The listing builds one solid part. Answer for the finished solid, in the listing's coordinates (mm). Give positions to 0.01 mm unless a question says otherwise; leave off trailing zeros. Order: outer loops, then holes, each group sorted by start corner. A loop starts at its lowest first (then second) coordinate and runs counter-clockwise, first axis right, second up. Notation, with made-up numbers: (75.25, -17.75) - (83.25, -17.75) arc R28 ccw to (83.25, 1.25) - close; hole circle Ø10 at (-24, -29.5). An arc over 180 degrees is marked (long way). Answer in a Markdown table with one row per item.
from build123d import *

# Parameters (mm, degrees)
SKETCH1_W           = 145
SKETCH1_H           = 68
BOSS_EXTRUDE1_DEPTH = 2
SKETCH2_R           = 1.65
SKETCH2_R_2         = 3
SKETCH2_R_3         = 1.1
CUT_EXTRUDE1_DEPTH  = 81.101498113


with BuildPart() as part:
    # Sketch1 → Boss-Extrude1 (new body)
    with BuildSketch(Plane.XY):
        Rectangle(SKETCH1_W, SKETCH1_H)
    extrude(amount=BOSS_EXTRUDE1_DEPTH)

    # Sketch2 → Cut-Extrude1 (cut, through all)
    with BuildSketch(Plane.XY.offset(2)):
        with Locations((53, 20)):
            Circle(SKETCH2_R)
        with Locations((53, -20)):
            Circle(SKETCH2_R)
        with Locations((-59.5, 15)):
            Circle(SKETCH2_R_2)
        with Locations((-59.5, -15)):
            Circle(SKETCH2_R_2)
        with Locations((-59.5, 0)):
            Circle(SKETCH2_R_3)
        with BuildLine():
            Line((61.5, -13.5), (44.5, -13.5))
            ThreePointArc((44.5, -13.5), (43.792893219, -13.207106781), (43.5, -12.5))
            Line((43.5, -12.5), (43.5, 12.5))
            ThreePointArc((43.5, 12.5), (43.792893219, 13.207106781), (44.5, 13.5))
            Line((44.5, 13.5), (61.5, 13.5))
            ThreePointArc((61.5, 13.5), (62.207106781, 13.207106781), (62.5, 12.5))
            Line((62.5, 12.5), (62.5, -12.5))
            ThreePointArc((62.5, -12.5), (62.207106781, -13.207106781), (61.5, -13.5))
        make_face()
    extrude(amount=-CUT_EXTRUDE1_DEPTH, mode=Mode.SUBTRACT)


solid = part.part
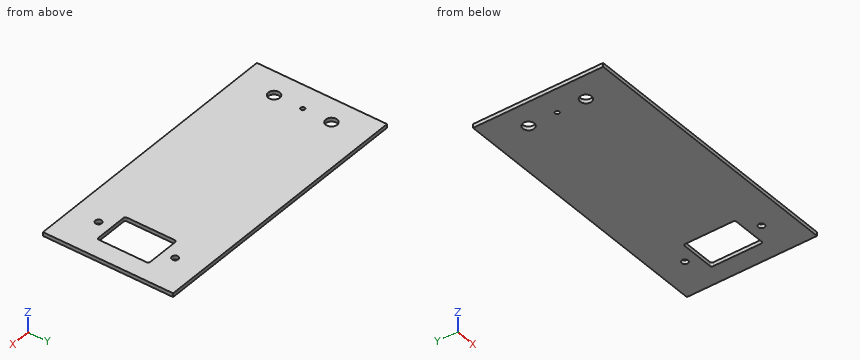
Item 1: Find section A-A on y = -9. Write down the section's boundary in (x, z).
Answer block:
| item | result |
|---|---|
| outline | (-72.5, 0) - (43.5, 0) - (43.5, 2) - (-72.5, 2) - close; (62.5, 0) - (72.5, 0) - (72.5, 2) - (62.5, 2) - close |
Item 2: This flat-tipped pin is pushed along its axis until it touches: P1, Ø5.5, axis at x = -59.5, y = 15, coming from the +Z side. Where does it stop, or does it pass through?
Answer block:
| item | result |
|---|---|
| P1 | through |
Item 3: Find section B-B on x = 53. Write down the section's boundary in (y, z), then the cut area to 3 significant figures.
Answer block:
| item | result |
|---|---|
| outline | (-34, 0) - (-21.65, 0) - (-21.65, 2) - (-34, 2) - close; (-18.35, 0) - (-13.5, 0) - (-13.5, 2) - (-18.35, 2) - close; (13.5, 0) - (18.35, 0) - (18.35, 2) - (13.5, 2) - close; (21.65, 0) - (34, 0) - (34, 2) - (21.65, 2) - close |
| area | 68.8 mm² |
Item 4: Find section C-C on y = -20. Write down the section's boundary in (x, z), then the cut area to 3 significant figures.
Answer block:
| item | result |
|---|---|
| outline | (-72.5, 0) - (51.35, 0) - (51.35, 2) - (-72.5, 2) - close; (54.65, 0) - (72.5, 0) - (72.5, 2) - (54.65, 2) - close |
| area | 283 mm² |
Item 5: Consider line 1 (Y direction, x = 53, z = 0.95); line 2 (Y direction, x = -59.5, z = 0.5); line 3 (X direction, y = -10.5, z = 0.4). Determine where each line is inside the solid, lowest interval first.
Answer block:
| item | result |
|---|---|
| line 1 | -34 to -21.65, -18.35 to -13.5, 13.5 to 18.35, 21.65 to 34 |
| line 2 | -34 to -18, -12 to -1.1, 1.1 to 12, 18 to 34 |
| line 3 | -72.5 to 43.5, 62.5 to 72.5 |
